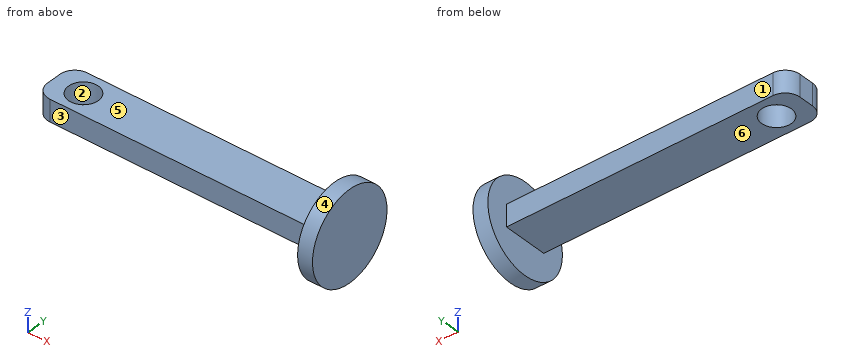
```python
from build123d import *

# Parameters (mm, degrees)
SKETCH1_R           = 9.525
BOSS_EXTRUDE1_DEPTH = 3.175
SKETCH2_W           = 4.6355
SKETCH2_H           = 9.525
BOSS_EXTRUDE2_DEPTH = 60
FILLET1_R           = 3.175
SKETCH3_R           = 3.175
CUT_EXTRUDE1_DEPTH  = 62.894881473


with BuildPart() as part:
    # Sketch1 → Boss-Extrude1 (new body)
    with BuildSketch(Plane(origin=(0, 0, 0), x_dir=(0, 0, -1), z_dir=(1, 0, 0))):
        Circle(SKETCH1_R)
    extrude(amount=BOSS_EXTRUDE1_DEPTH)

    # Sketch2 → Boss-Extrude2 (add)
    with BuildSketch(Plane.ZY):
        Rectangle(SKETCH2_W, SKETCH2_H)
    extrude(amount=BOSS_EXTRUDE2_DEPTH)

    # Fillet1
    fillet1_edges = [part.edges().sort_by_distance(p)[0] for p in [
        (-60, 4.7625, 0),
        (-60, -4.7625, 0),
    ]]
    fillet(fillet1_edges, radius=FILLET1_R)

    # Sketch3 → Cut-Extrude1 (cut, through all)
    with BuildSketch(Plane(origin=(0, 0, -2.31775), x_dir=(-1, 0, 0), z_dir=(0, 0, -1))):
        with Locations(Location((53.65, 0, 0), (0, 0, 90))):
            Circle(SKETCH3_R)
    extrude(amount=-CUT_EXTRUDE1_DEPTH, mode=Mode.SUBTRACT)


solid = part.part
```
Check sheet for the modelled part. Datum: model origin and axes. Units: mm. Face numbers are marked on the shaded views. A direction names the side the tool comes from. Round coordinates to 2 decimals unless told otherwise and drop trailing zeros. Write each loop counter-clockwise with the first axis right and the second up, starting at its lowest first coordinate (ties: lowest second). Pieces come first, ordered by that corner, then holes. Notation, with made-up numbers: (-11, -30) -> (25, -30) arc R16 ccw to (25, -11) -> close; hole circle Ø9 at (85, 4.5). An arc over 180 degrees is marked (long way). One line per question, with ' | ' between items. Start each with the question number.
1. Release check for a two-part mould opening along Y. For the marked faces 1, 2 and 3 record: +Y half, -Y half, draft (parallel to the pull), parting line (faces both ways), or undercut.
2. Depth check by flat-ended pin: pin 1 (4 mm diameter, centred on x = -39, z = 0.5, fed in from +Y); pin 2 (1.5 mm diameter, centred on y = 3, z = 5.5, fed in from -X); pin 3 (5.5 mm diameter, centred on y = 3, z = 3.5, fed in from -X); pin 4 (4 mm diameter, centred on x = -44, y = 5.5, fed in from +Z). Enter the tip coordinate at first touch or a pass-through.
3. Sectioned sample at B-B, the plane y = 0. Record the cut outline in (x, z) (3 decimals), then the cut area to 3 significant figures.
4. Sectioned sample at A-A, the plane x = -53.65. Record the cut outline in (y, z) (1 decimal).
5. Sectioned sample at D-D, the plane x = -14.5. Record the cut outline in (y, z).
6. Scan lines: line 1 along X through (y, z) = (0, -0.9) (3 decimals); line 2 along X through (y, z) = (-2.5, 7.75) (3 decimals); line 3 along Z through (x, y) = (-19, 4). Record each from-to range of solid material in increasing order. Write a range as from..to.
7. Set-up check for the marked faces 4, 5 and 6: record each of +Z, -Z, +X, -X, +Y, -Y from which the full face is reachable in a straight line by a thin tool's end or side.
Taken from the geometry:
1) face 1: +Y half | face 2: undercut | face 3: -Y half
2) pin 1: stops at y = 4.76 | pin 2: stops at x = 0 | pin 3: stops at x = -60 | pin 4: stops at z = 2.32
3) outline: (-60, -2.318) -> (-56.825, -2.318) -> (-56.825, 2.318) -> (-60, 2.318) -> close; (-50.475, -2.318) -> (0, -2.318) -> (0, -9.525) -> (3.175, -9.525) -> (3.175, 9.525) -> (0, 9.525) -> (0, 2.318) -> (-50.475, 2.318) -> close | area: 309 mm^2
4) outline: (-4.8, -2.3) -> (-3.2, -2.3) -> (-3.2, 2.3) -> (-4.8, 2.3) -> close; (3.2, -2.3) -> (4.8, -2.3) -> (4.8, 2.3) -> (3.2, 2.3) -> close
5) outline: (-4.76, -2.32) -> (4.76, -2.32) -> (4.76, 2.32) -> (-4.76, 2.32) -> close
6) line 1: x = -60..-56.825, -50.475..3.175 | line 2: x = 0..3.175 | line 3: z = -2.32..2.32
7) face 4: +X, -X | face 5: +Z, -X, +Y, -Y | face 6: -Z, -X, +Y, -Y
